```python
from build123d import *

# Parameters (mm, degrees)
SKETCH1_R               = 12.7
EXTRUDE1_DEPTH          = 228.6
SKETCH2_R               = 5
EXTRUDE2_DEPTH          = 2
SKETCH3_R               = 13.7
EXTRUDE3_DEPTH          = 4
SKETCH4_R               = 4
EXTRUDE4_DEPTH          = 7
SKETCH5_W               = 127.127972269
SKETCH5_H               = 9.602426348
CUT_EXTRUDE1_DEPTH      = 14.7
CUT_EXTRUDE1_DEPTH_BACK = 14.7


with BuildPart() as part:
    # Sketch1 → Extrude1 (new body)
    with BuildSketch(Plane(origin=(0, 0, 0), x_dir=(0, 0, -1), z_dir=(1, 0, 0))):
        Circle(SKETCH1_R)
    extrude(amount=EXTRUDE1_DEPTH)

    # Sketch2 → Extrude2 (add, symmetric)
    with BuildSketch(Plane.XY):
        with BuildLine():
            Line((0, 7.778067586), (-23.625125491, 7.778067586))
            ThreePointArc((-23.625125491, 7.778067586), (-31.403193077, 0), (-23.625125491, -7.778067586))
            Line((-23.625125491, -7.778067586), (0, -7.778067586))
            Line((0, -7.778067586), (0, 7.778067586))
        make_face()
        with Locations((-23.625125491, 0)):
            Circle(SKETCH2_R, mode=Mode.SUBTRACT)
    extrude(amount=EXTRUDE2_DEPTH, both=True)

    # Sketch3 → Extrude3 (add)
    with BuildSketch(Plane(origin=(228.6, 0, 0), x_dir=(0, 0, -1), z_dir=(1, 0, 0))):
        Circle(SKETCH3_R)
    extrude(amount=EXTRUDE3_DEPTH)

    # Sketch4 → Extrude4 (add, symmetric)
    with BuildSketch(Plane.XY):
        with BuildLine():
            Line((232.6, 10.132851916), (253.6, 10.132851916))
            ThreePointArc((253.6, 10.132851916), (263.732851916, 0), (253.6, -10.132851916))
            Line((253.6, -10.132851916), (232.6, -10.132851916))
            Line((232.6, -10.132851916), (232.6, 10.132851916))
        make_face()
        with Locations((253.6, 0)):
            Circle(SKETCH4_R, mode=Mode.SUBTRACT)
    extrude(amount=EXTRUDE4_DEPTH, both=True)

    # Sketch5 → Cut-Extrude1 (cut, two sides)
    with BuildSketch(Plane(origin=(0, 0, 0), x_dir=(1, 0, 0), z_dir=(0, 1, 0))) as cut_extrude1_sk:
        with Locations((296.163986135, 0)):
            Rectangle(SKETCH5_W, SKETCH5_H)
    extrude(amount=CUT_EXTRUDE1_DEPTH, mode=Mode.SUBTRACT)
    extrude(cut_extrude1_sk.sketch, amount=-CUT_EXTRUDE1_DEPTH_BACK, mode=Mode.SUBTRACT)


solid = part.part
```
Work out the finished part from the listing and answer in its coordinate system (mm). A direction names the side the tool comes from. Coordinates: 2 decimals unless noted, no trailing zeros. Loops run counter-clockwise (first coordinate to the right, second up) from the corner with the lowest first, then second, coordinate; pieces in that order, holes last. Notation, with made-up numbers: M 7,89.5 L 30,89.5 A22 ccw 30,123.5 Z; hole C 56,4.5 d10. An arc over 180 degrees is marked long. Use CSV: the item, a comma, the result in double quotes. Start each with the question number.
(1) Consider line 1 (Z direction, x = 242, y = -0.5); line 2 (X direction, y = 0, z = -5.4); line 3 (Y direction, x = 253.6, z = 6.05). Determine where each line is inside the solid, lowest interval first.
(2) Find section A-A, the plane y = 0. State how many separate pieces and enclosed holes the cut face has, then the cut area to 3 significant figures.
(3) Given pin 1 Ø8 at (x, y) = (-23.63, 0) entering from -Z; pin 2 Ø1 at (y, z) = (9.5, 6) entering from +X; pin 3 Ø6 at (x, y) = (158, 0.5) entering from -Z; pin 4 Ø1.5 at (x, z) = (62, -3.5) entering from -Y, each flat-ended and moving along its own axis, determine where each tip first touches the part or whether it passes through.
(4) For a pull along Y with two mould halves and no side action, classify faces 4 (the face through (-12, 0, 2)), 5 (the face through (263.73, 0.22, -5.89)), 6 (the face through (249.604, 0.176, 5.885)) as +Y half, -Y half, draft (parallel to the pull), parting line (faces both ways), or undercut.
(5) For faces 1 (the face through (248, 0, 7)), 2 (the face through (228.6, -9.1, -9.1)), 3 (the face through (248, 0, -7)), determine the directions among +Z, -Z, +X, -X, +Y, -Y from which every point of the face is accessible in a straight line to the end or side of a thin tool.
(6) Find section B-B, the plane x = 92.5. Give the vertices of the cut face in (y, z).
Recorded:
1,line 1,"z = -7 to -4.8, 4.8 to 7"
1,line 2,"x = 0 to 249.6, 257.6 to 263.73"
1,line 3,"y = -10.13 to -4, 4 to 10.13"
2,separate pieces,"4"
2,enclosed holes,"0"
2,area,"6,100 mm^2"
3,pin 1,"passes through"
3,pin 2,"stops at x = 258.26"
3,pin 3,"stops at z = -12.7"
3,pin 4,"stops at y = -12.4"
4,face 4,"draft"
4,face 5,"parting line"
4,face 6,"undercut"
5,face 1,"+Z, +X, +Y, -Y"
5,face 2,"-X"
5,face 3,"-Z, +X, +Y, -Y"
6,outline,"C 0,0 d25.4"
